Could you check a few things on this drawing? It's one solid part, dimensions in mm from its lowest x, y, z. A direction names the side the tool comes from. Coordinates: 2 decimals unless noted, no trailing zeros. Write each loop counter-clockwise with the first axis right and the second up, starting at its lowest first coordinate (ties: lowest second). Pieces come first, ordered by that corner, then holes. Notation, with made-up numbers: M 60,19 L 85,19 A6 cw 85,28 Z; hole C -2.75,54 d1. An arc over 180 degrees is marked long. Use a Markdown table: item, result.
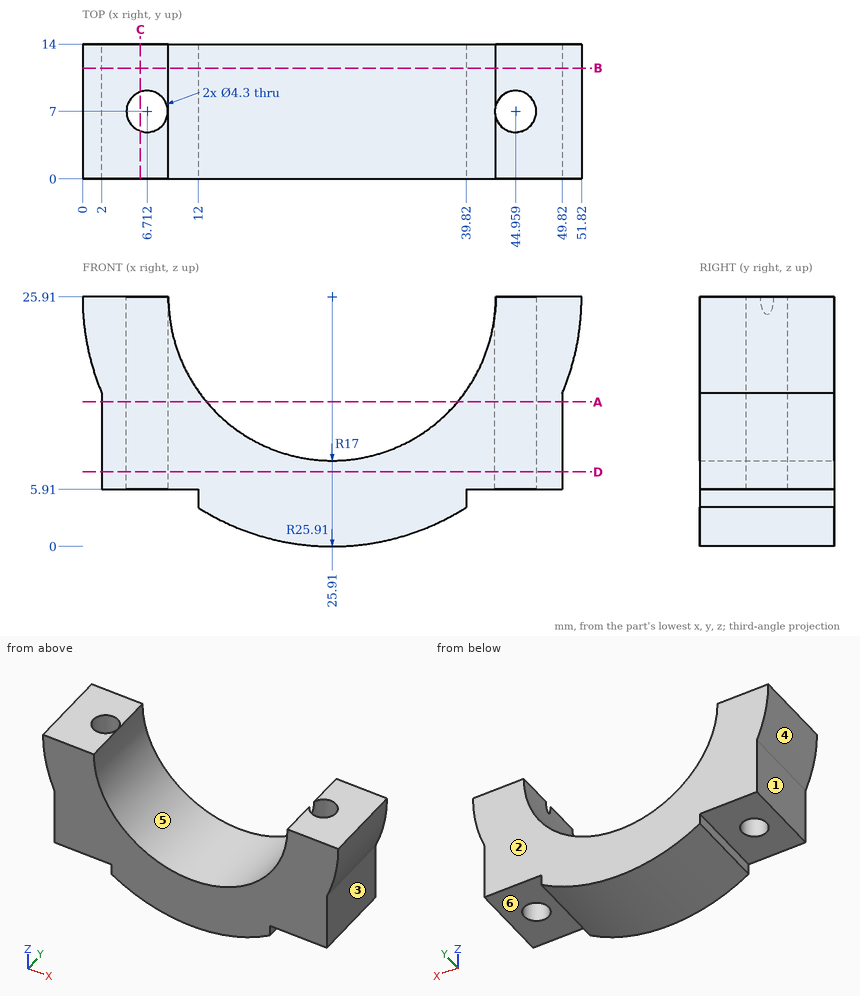
1. Suppose I cut it at C-C on x = 6. Write out the boundary of the cut face in (y, z).
Answers follow:
| item | result |
|---|---|
| outline | M 0,5.91 L 4.97,5.91 L 4.97,25.91 L 0,25.91 Z; M 9.03,5.91 L 14,5.91 L 14,25.91 L 9.03,25.91 Z |
2. Which directions (+Z, -Z, +X, -X, +Y, -Y) give clear straight access to the entire face, cutting with the end or side of a thin tool? Please do the marked faces 1, 2 and 3.
Answers follow:
| item | result |
|---|---|
| face 1 | -Z, -X, +Y, -Y |
| face 2 | +Z, -Z, +X, -X, +Y |
| face 3 | -Z, +X, +Y, -Y |
3. Will these pins go through, and if not, where does the flat tip stop? pin 1 Ø0.6 at (y, z) = (9, 4.5) entering from +X; pin 2 Ø3 at (y, z) = (7.5, 9) entering from -X; pin 3 Ø3.5 at (x, y) = (44.96, 7) entering from +Z; pin 4 Ø3 at (x, y) = (8, 9) entering from -Z.
Answers follow:
| item | result |
|---|---|
| pin 1 | stops at x = 39.82 |
| pin 2 | stops at x = 2 |
| pin 3 | passes through |
| pin 4 | stops at z = 5.91 |
4. Suppose I cut it at D-D on z = 7.75. Write out the boundary of the cut face in (x, y).
Answers follow:
| item | result |
|---|---|
| outline | M 2,0 L 49.82,0 L 49.82,14 L 2,14 Z; hole C 6.71,7 d4.3; hole C 44.96,7 d4.3 |
5. Suppose I cut it at A-A on z = 15. Write out the boundary of the cut face in (x, y), and give its area (3 significant figures).
Answers follow:
| item | result |
|---|---|
| outline | M 2,0 L 12.87,0 L 12.87,14 L 2,14 Z; M 38.95,0 L 49.82,0 L 49.82,14 L 38.95,14 Z; hole C 6.71,7 d4.3; hole C 44.96,7 d4.3 |
| area | 275 mm2 |
6. We'd pull the mould along X, two halves only. Please class the marked faces 4, 5 and 6: +X half, -X half, draft (parallel to the pull), parting line (faces both ways), or undercut.
Answers follow:
| item | result |
|---|---|
| face 4 | -X half |
| face 5 | undercut |
| face 6 | draft |
7. Suppose I cut it at B-B on y = 11.5. Write out the boundary of the cut face in (x, z).
Answers follow:
| item | result |
|---|---|
| outline | M 0,25.91 A25.91 ccw 2,15.93 L 2,5.91 L 12,5.91 L 12,4.05 A25.91 ccw 39.82,4.05 L 39.82,5.91 L 49.82,5.91 L 49.82,15.93 A25.91 ccw 51.82,25.91 L 42.91,25.91 A17 cw 8.91,25.91 Z |
8. I need wall thicknesses on probe 1 along Z at (x, y) = (47, 11); probe 2 along X at (y, z) = (5.25, 20.25) (1 decimal); probe 3 along X at (y, z) = (7.5, 12). Which ranges of each line are inside material? Lowest first, please.
Answers follow:
| item | result |
|---|---|
| probe 1 | z = 5.91 to 25.91 |
| probe 2 | x = 0.6 to 5.5, 8 to 9.9, 41.9 to 43.7, 46.2 to 51.2 |
| probe 3 | x = 2 to 4.62, 8.8 to 16.14, 35.68 to 42.87, 47.05 to 49.82 |
